Model file for the job. Use its own axes, mm. A direction names the side the tool comes from. Round coordinates to 2 decimals unless told otherwise and drop trailing zeros. Loops run counter-clockwise (first coordinate to the right, second up) from the corner with the lowest first, then second, coordinate; pieces in that order, holes last. Notation, with made-up numbers: (-37, 53) - (22, 53) arc R29 ccw to (22, 80) - close; hole circle Ø7 at (32.25, 3.25). An arc over 180 degrees is marked (long way). Answer as a JSON object with one key per item and string values.
Autodesk Inventor part; units mm, degrees
ref_plane "YZ Plane" through (0, 0, 0) normal (1, 0, 0) x (0, 1, 0)
ref_plane "XZ Plane" through (0, 0, 0) normal (0, 1, 0) x (-1, 0, 0)
ref_plane "XY Plane" through (0, 0, 0) normal (0, 0, 1) x (1, 0, 0)
sketch "Skizze1" plane through (0, 0, 0) normal (0, 0, 1) x (1, 0, 0)
  line L0 (-29.4, 0) -> (29.4, 0) construction
  circle A0 centre (0, 0) radius 16.6 construction
  line L1 (0, 0) -> (-14.376, -8.3) construction
  line L2 (0, 0) -> (14.376, -8.3) construction
  line L3 (0, 29.4) -> (0, -29.4) construction
  line L4 (0, 0) -> (0, 16.6) construction
  circle A1 centre (0, 0) radius 9.75
  circle A2 centre (0, 0) radius 20
  circle A3 centre (0, 0) radius 6.35 construction
  circle A4 centre (-6.35, 0) radius 1.65
  circle A5 centre (0, 6.35) radius 1.65
  circle A6 centre (6.35, 0) radius 1.65
  circle A7 centre (0, -6.35) radius 1.65
  circle A8 centre (0, 0) radius 21
  circle A9 centre (0, 0) radius 21
  circle A10 centre (-14.376, -8.3) radius 2.45
  circle A11 centre (0, 16.6) radius 2.45
  circle A12 centre (14.376, -8.3) radius 2.45
  circle A13 centre (0, 0) radius 19
  circle A14 centre (0, 0) radius 4
  dimension "d1" = 33.2
  dimension "d2" = 120
  dimension "d13" = 120
  dimension "d14" = 19.5
  dimension "d16" = 40
  dimension "d21" = 6.35
  dimension "d22" = 3.3
  dimension "d26" = 1
  dimension "d27" = 1
  dimension "d30" = 4.9
  dimension "d33" = 1
  dimension "d42" = 8
extrude "Extrusion1" add sketch "Skizze1" along normal blind 1 contours A1 | A2 | A4 | A5 | A6 | A7 | A8 | A10 A13 | A10 A13 A11 A12 | A13 A10 | A13 A11 | A11 A13 | A13 A12 | A12 A13 | A14
extrude "Extrusion3" add sketch "Skizze1" along normal blind 7 from surface at 1 contours A1 | A2 | A4 | A5 | A6 | A7 | A10 A13 | A10 A13 A11 A12 | A13 A10 | A13 A11 | A11 A13 | A13 A12 | A12 A13 | A14
extrude "Extrusion8" add sketch "Skizze1" along normal blind 16 from surface at 8 contours A10 A13 | A13 A10 | A13 A11 | A11 A13 | A13 A12 | A12 A13
extrude "Extrusion9" cut sketch "Skizze1" along normal blind 5 contours A1 | A4 | A5 | A6 | A7 | A14
extrude "Extrusion10" cut sketch "Skizze1" along normal through all contours A4 | A5 | A6 | A7 | A14
extrude "Extrusion11" cut sketch "Skizze1" against normal blind 0.5 from surface at 8 contours A1 | A4 | A5 | A6 | A7 | A14
equation "\"d13\" = d2"
properties part number "Output"
1) Two-plate mould, pull along Y, no slides. Class faces 1 (the cylindrical face through (-0.32, 14.17, 15.89)), 2 (the flat face through (9, 5, 8)), 3 (the cylindrical face through (-1.269, -9.667, 2.465)): pulls with the +Y half, pulls with the -Y half, needs draft (parallel to the pull), parting line crosses it, or undercut.
Values follow:
{"face 1": "parting line crosses it", "face 2": "needs draft", "face 3": "undercut"}
2) Probe probe 1 along Y at (x, z) = (0, 7.75); probe 2 along Y at (x, z) = (0.5, 5.25); probe 3 along Z at (x, y) = (-2.5, -11.5). List the from-to ranges inside material, lowest first.
Values follow:
{"probe 1": "-20 to -9.75, 9.75 to 20", "probe 2": "-19.99 to -7.92, -4.78 to -3.97, 3.97 to 4.78, 7.92 to 19.99", "probe 3": "0 to 8"}
3) Slice it at A-A on x = 0. Count the separate pieces of the cut face and the enclosed holes in it, then the cut area to 3 significant figures.
Values follow:
{"separate pieces": "4", "enclosed holes": "0", "area": "257 mm²"}
4) Slice it at C-C on z = 6.75. List the corners of the cut face in (x, y).
Values follow:
{"outline": "circle Ø40 at (0, 0); hole circle Ø3.3 at (-6.35, 0); hole circle Ø8 at (0, 0); hole circle Ø3.3 at (0, -6.35); hole circle Ø3.3 at (0, 6.35); hole circle Ø3.3 at (6.35, 0)"}
5) Drop flat-ended pins along their axis: P1, Ø10, axis at x = 12, y = -16, coming from the +Z side; P2, Ø17.5, axis at x = 0, y = 0, coming from the +Z side; P3, Ø2, axis at x = 6.35, y = 0, coming from the +Z side; P4, Ø10, axis at x = -3.5, y = -3.5, coming from the -Z side. Give the stop position or say it passes through.
Values follow:
{"P1": "z = 8", "P2": "z = 7.5", "P3": "through", "P4": "z = 0"}
6) Slice it at B-B on y = 0. List the corners of the cut face in (x, z).
Values follow:
{"outline": "(-21, 0) - (-9.75, 0) - (-9.75, 5) - (-8, 5) - (-8, 7.5) - (-9.75, 7.5) - (-9.75, 8) - (-20, 8) - (-20, 1) - (-21, 1) - close; (-4.7, 5) - (-4, 5) - (-4, 7.5) - (-4.7, 7.5) - close; (4, 5) - (4.7, 5) - (4.7, 7.5) - (4, 7.5) - close; (8, 5) - (9.75, 5) - (9.75, 0) - (21, 0) - (21, 1) - (20, 1) - (20, 8) - (9.75, 8) - (9.75, 7.5) - (8, 7.5) - close"}
7) Tool access for faces 4 (the flat face through (4.2, 0.1, 5)), 5 (the cylindrical face through (-4.826, 0.632, 6.232)), 6 (the cylindrical face through (-4.336, 19.524, 4.451)): list every direction of +Z, -Z, +X, -X, +Y, -Y with a clear straight run to the whole face (end or side of a thin tool).
Values follow:
{"face 4": "-Z", "face 5": "+Z, -Z", "face 6": "+Z"}
8) Slice it at D-D on z = 9.5. List the corners of the cut face in (x, y).
Values follow:
{"outline": "circle Ø4.9 at (-14.38, -8.3); circle Ø4.9 at (0, 16.6); circle Ø4.9 at (14.38, -8.3)"}
